Autodesk Inventor part; units mm, degrees
ref_plane "side_4d_XY" through (-20, 0, -165) normal (-1, 0, 0) x (0, 1, 0)
ref_plane "side_4d_YZ" through (-20, 0, -165) normal (0, 1, 0) x (0, 0, -1)
ref_plane "side_4d_ZX" through (-20, 0, -165) normal (0, 0, -1) x (-1, 0, 0)
sketch "Skizze_1" plane through (0, 0, 0) normal (0, 0, 1) x (1, 0, 0)
  arc A0 (-20, -17) -> (-17, -20) centre (-17, -17) ccw
  line L0 (-17, -20) -> (-4.1, -20)
  line L1 (-4.1, -20) -> (-4.1, -17)
  line L2 (-4.1, -17) -> (-10.5, -17)
  line L3 (-10.5, -17) -> (-10.5, -13.6627)
  arc A1 (-10.0314, -12.5314) -> (-10.5, -13.6627) centre (-8.9002, -13.6627) ccw
  line L4 (-10.0314, -12.5314) -> (-7.4645, -9.9645)
  arc A2 (-3.9289, -8.5) -> (-7.4645, -9.9645) centre (-3.9289, -13.5) ccw
  line L5 (-3.9289, -8.5) -> (3.9289, -8.5)
  arc A3 (7.4645, -9.9645) -> (3.9289, -8.5) centre (3.9289, -13.5) ccw
  line L6 (7.4645, -9.9645) -> (10.0314, -12.5314)
  arc A4 (10.5, -13.6627) -> (10.0314, -12.5314) centre (8.9002, -13.6627) ccw
  line L7 (10.5, -13.6627) -> (10.5, -17)
  line L8 (10.5, -17) -> (4.1, -17)
  line L9 (4.1, -17) -> (4.1, -20)
  line L10 (4.1, -20) -> (17, -20)
  arc A5 (17, -20) -> (20, -17) centre (17, -17) ccw
  line L11 (20, -17) -> (20, -4.1)
  line L12 (20, -4.1) -> (17, -4.1)
  line L13 (17, -4.1) -> (17, -10.5)
  line L14 (17, -10.5) -> (13.6627, -10.5)
  arc A6 (12.5314, -10.0314) -> (13.6627, -10.5) centre (13.6627, -8.9002) ccw
  line L15 (12.5314, -10.0314) -> (9.9645, -7.4645)
  arc A7 (8.5, -3.9289) -> (9.9645, -7.4645) centre (13.5, -3.9289) ccw
  line L16 (8.5, -3.9289) -> (8.5, 3.9289)
  arc A8 (9.9645, 7.4645) -> (8.5, 3.9289) centre (13.5, 3.9289) ccw
  line L17 (9.9645, 7.4645) -> (12.5314, 10.0314)
  arc A9 (13.6627, 10.5) -> (12.5314, 10.0314) centre (13.6627, 8.9002) ccw
  line L18 (13.6627, 10.5) -> (17, 10.5)
  line L19 (17, 10.5) -> (17, 4.1)
  line L20 (17, 4.1) -> (20, 4.1)
  line L21 (20, 4.1) -> (20, 17)
  arc A10 (20, 17) -> (17, 20) centre (17, 17) ccw
  line L22 (17, 20) -> (4.1, 20)
  line L23 (4.1, 20) -> (4.1, 17)
  line L24 (4.1, 17) -> (10.5, 17)
  line L25 (10.5, 17) -> (10.5, 13.6627)
  arc A11 (10.0314, 12.5314) -> (10.5, 13.6627) centre (8.9002, 13.6627) ccw
  line L26 (10.0314, 12.5314) -> (7.4645, 9.9645)
  arc A12 (3.9289, 8.5) -> (7.4645, 9.9645) centre (3.9289, 13.5) ccw
  line L27 (3.9289, 8.5) -> (-3.9289, 8.5)
  arc A13 (-7.4645, 9.9645) -> (-3.9289, 8.5) centre (-3.9289, 13.5) ccw
  line L28 (-7.4645, 9.9645) -> (-10.0314, 12.5314)
  arc A14 (-10.5, 13.6627) -> (-10.0314, 12.5314) centre (-8.9002, 13.6627) ccw
  line L29 (-10.5, 13.6627) -> (-10.5, 17)
  line L30 (-10.5, 17) -> (-4.1, 17)
  line L31 (-4.1, 17) -> (-4.1, 20)
  line L32 (-4.1, 20) -> (-17, 20)
  arc A15 (-17, 20) -> (-20, 17) centre (-17, 17) ccw
  line L33 (-20, 17) -> (-20, 4.1)
  line L34 (-20, 4.1) -> (-17, 4.1)
  line L35 (-17, 4.1) -> (-17, 10.5)
  line L36 (-17, 10.5) -> (-13.6627, 10.5)
  arc A16 (-12.5314, 10.0314) -> (-13.6627, 10.5) centre (-13.6627, 8.9002) ccw
  line L37 (-12.5314, 10.0314) -> (-9.9645, 7.4645)
  arc A17 (-8.5, 3.9289) -> (-9.9645, 7.4645) centre (-13.5, 3.9289) ccw
  line L38 (-8.5, 3.9289) -> (-8.5, -3.9289)
  arc A18 (-9.9645, -7.4645) -> (-8.5, -3.9289) centre (-13.5, -3.9289) ccw
  line L39 (-9.9645, -7.4645) -> (-12.5314, -10.0314)
  arc A19 (-13.6627, -10.5) -> (-12.5314, -10.0314) centre (-13.6627, -8.9002) ccw
  line L40 (-13.6627, -10.5) -> (-17, -10.5)
  line L41 (-17, -10.5) -> (-17, -4.1)
  line L42 (-17, -4.1) -> (-20, -4.1)
  line L43 (-20, -4.1) -> (-20, -17)
  circle A20 centre (0, 0) radius 6
extrude "Extrusion1" add sketch "Skizze_1" against normal blind 160
sketch "Sketch2" plane through (0, 0, 0) normal (0, 0, 1) x (1, 0, 0)
  point P0 (-15, -15)
hole "Drilling 1" at (-15, -15, 0) direction (0, 0, -1) diameter 5 depth 6000
sketch "Sketch3" plane through (0, 0, 0) normal (0, 0, 1) x (1, 0, 0)
  point P0 (15, -15)
hole "Drilling 2" at (15, -15, 0) direction (0, 0, -1) diameter 5 depth 6000
sketch "Sketch4" plane through (0, 0, 0) normal (0, 0, 1) x (1, 0, 0)
  point P0 (15, 15)
hole "Drilling 3" at (15, 15, 0) direction (0, 0, -1) diameter 5 depth 6000
sketch "Sketch5" plane through (0, 0, 0) normal (0, 0, 1) x (1, 0, 0)
  point P0 (-15, 15)
hole "Drilling 4" at (-15, 15, 0) direction (0, 0, -1) diameter 5 depth 6000
ref_plane "side_4d_XY" through (-20, 0, -165) normal (-1, 0, 0) x (0, 1, 0)
ref_plane "side_4d_YZ" through (-20, 0, -165) normal (0, 1, 0) x (0, 0, -1)
ref_plane "side_4d_ZX" through (-20, 0, -165) normal (0, 0, -1) x (-1, 0, 0)
ref_plane "side_1a_XY" through (0, 20, -165) normal (0, 1, 0) x (1, 0, 0)
ref_plane "side_1a_YZ" through (0, 20, -165) normal (1, 0, 0) x (0, 0, -1)
ref_plane "side_1a_ZX" through (0, 20, -165) normal (0, 0, -1) x (0, 1, 0)
ref_plane "side_2b_XY" through (20, 0, -165) normal (1, 0, 0) x (0, -1, 0)
ref_plane "side_2b_YZ" through (20, 0, -165) normal (0, -1, 0) x (0, 0, -1)
ref_plane "side_2b_ZX" through (20, 0, -165) normal (0, 0, -1) x (1, 0, 0)
ref_plane "side_3c_XY" through (0, -20, -165) normal (0, -1, 0) x (-1, 0, 0)
ref_plane "side_3c_YZ" through (0, -20, -165) normal (-1, 0, 0) x (0, 0, -1)
ref_plane "side_3c_ZX" through (0, -20, -165) normal (0, 0, -1) x (0, -1, 0)
ref_plane "end_XY" through (0, 0, -330) normal (0, 0, -1) x (1, 0, 0)
ref_plane "end_YZ" through (0, 0, -330) normal (1, 0, 0) x (0, -1, 0)
ref_plane "end_ZX" through (0, 0, -330) normal (0, -1, 0) x (0, 0, -1)
ref_plane "start_XY" through (0, 0, 0) normal (0, 0, 1) x (1, 0, 0)
ref_plane "start_YZ" through (0, 0, 0) normal (1, 0, 0) x (0, 1, 0)
ref_plane "start_ZX" through (0, 0, 0) normal (0, 1, 0) x (0, 0, 1)
properties part number "MayTec 1_11_040040_43S_Profile 40x40, 4E, S_160_Detail_(0;0,0,0)"
Input: part model. Units: mm. Frame: model coordinates. A direction names the side the tool comes from. Round coordinates to 2 decimals unless told otherwise and drop trailing zeros. Order: outer loops, then holes, each group sorted by start corner. A loop starts at its lowest first (then second) coordinate and runs counter-clockwise, first axis right, second up. Notation, with made-up numbers: (86, 67.5) - (108, 67.5) arc R16 ccw to (108, 78.5) - close; hole circle Ø7 at (-29.75, 9). An arc over 180 degrees is marked (long way). One line per question, with ' | ' between items. Start each with the question number.
1) Contact query for flat-ended pins moving along their axis: P1, Ø3.5, axis at y = 19, z = -93, coming from the +X side; P2, Ø0.9, axis at y = -18.5, z = -65, coming from the +X side; P3, Ø2.5, axis at y = 0, z = -115.5, coming from the -X side. Output: stop coordinate, or through.
2) Pull-direction query (Y, two-part tool) for faces 1 (the flat face through (-11, -20, -79)), 2 (the flat face through (-4.1, 18, -79)), 3 (the cylindrical face through (-8.87, 5.82, -78.88)); classes: +Y half, -Y half, draft (parallel to the pull), parting line (faces both ways), or undercut.
3) Set-up query: faces 4 (the flat face through (20, -11, -79)), 5 (the flat face through (0, 8.5, -79)), 6 (the flat face through (-19, 4.1, -79)), 7 (the flat face through (7, -17, -79)), 8 (the cylindrical face through (19.1, -19.14, -78.88)). Return all of +Z, -Z, +X, -X, +Y, -Y with unobstructed straight access to the full face (end or side cutting, diameter ignored); none if empty.
4) Cut plane B-B, the plane z = -22.5. Give the number of separate pieces and of enclosed holes in the cut face, then the cut area to 3 significant figures.
5) Cut plane A-A, the plane y = 0. Return the cut outline in (x, z), then the cut area to 3 significant figures.
6) Ray query, probe 1 along Y at (x, z) = (15, -47); probe 2 along Y at (x, z) = (7.5, -89). Return the intervals inside material, ascending.
Worked out:
1) P1: stops at x = 19.99 | P2: stops at x = 19.81 | P3: stops at x = -8.5
2) face 1: -Y half | face 2: draft | face 3: undercut
3) face 4: +Z, -Z, +X, +Y, -Y | face 5: +Z, -Z, +Y | face 6: +Z, -Z, -X | face 7: +Z, -Z | face 8: +Z, -Z, +X, -Y
4) separate pieces: 1 | enclosed holes: 5 | area: 674 mm^2
5) outline: (-8.5, -160) - (-6, -160) - (-6, 0) - (-8.5, 0) - close; (6, -160) - (8.5, -160) - (8.5, 0) - (6, 0) - close | area: 800 mm^2
6) probe 1: y = -20 to -17.5, -12.5 to -10.5, 10.5 to 12.5, 17.5 to 20 | probe 2: y = -20 to -17, -10 to 10, 17 to 20
